CAD build for the part. Positions are in the model's coordinates, mm. Round coordinates to 2 decimals unless told otherwise and drop trailing zeros. Loops run counter-clockwise (first coordinate to the right, second up) from the corner with the lowest first, then second, coordinate; pieces in that order, holes last. Notation, with made-up numbers: M 41.25,27 L 81.25,27 A24 cw 81.25,37 Z; hole C 63.5,14 d10. An arc over 180 degrees is marked long. Use a Markdown table: item, result. Add a question column.
(1) Wall check: L1, parallel to Y at x = -8, z = 41; L2, parallel to Y at x = -8, z = 142.5; L3, parallel to X at y = -6, z = 482. Give the ranges that are in metal, low to high.
(2) Flat gauge pin, fed straight in: P1, Ø3, axis at x = 2, z = 545, coming from the +Y side. Where does the tip first touch, or does it go through?
(3) Band-saw the part on A-A, the plane z = 437.5. Write the cut outline in (x, y), and give its area (3 significant figures).
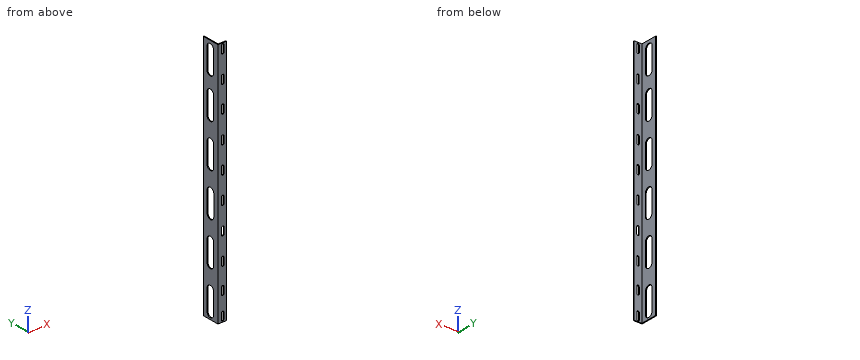
from build123d import *

# Parameters (mm, degrees)
BOSS_EXTRUDE1_DEPTH = 705
CUT_EXTRUDE2_DEPTH  = 10
CUT_EXTRUDE3_DEPTH  = 10


with BuildPart() as part:
    # Sketch1 → Boss-Extrude1 (new body)
    with BuildSketch(Plane.XY):
        Polygon((-9.451520251, 23.80952381), (-9.451520251, -26.19047619), (15.548479749, -26.19047619), (15.548479749, -23.69047619), (-6.951520251, -23.69047619), (-6.951520251, 23.80952381), align=None)
    extrude(amount=BOSS_EXTRUDE1_DEPTH)

    # Sketch3 → Cut-Extrude2 (cut)
    with BuildSketch(Plane(origin=(0, -23.69047619, 0), x_dir=(1, 0, 0), z_dir=(0, 1, 0))):
        with BuildLine():
            Line((1.100010518, -238.921557585), (1.100010518, -219.921557585))
            ThreePointArc((1.100010518, -219.921557585), (4.600010518, -217.057732255), (8.100010518, -219.921557585))
            Line((8.100010518, -219.921557585), (8.100010518, -238.921557585))
            ThreePointArc((8.100010518, -238.921557585), (4.600010518, -242.50349619), (1.100010518, -238.921557585))
        make_face()
        with BuildLine():
            Line((1.062751019, -162.814659823), (1.06366359, -143.814659845))
            ThreePointArc((1.06366359, -143.814659845), (4.564952106, -140.315948836), (8.063663115, -143.817237352))
            Line((8.063663115, -143.817237352), (8.064681771, -162.817237325))
            ThreePointArc((8.064681771, -162.817237325), (4.562374007, -166.462622847), (1.062751019, -162.814659823))
        make_face()
        with BuildLine():
            Line((0.583868221, -24.003598612), (0.583868221, -6.003598612))
            ThreePointArc((0.583868221, -6.003598612), (4.083868221, -2.503598612), (7.583868221, -6.003598612))
            Line((7.583868221, -6.003598612), (7.583868221, -24.003598612))
            ThreePointArc((7.583868221, -24.003598612), (4.083868221, -27.503598612), (0.583868221, -24.003598612))
        make_face()
        with BuildLine():
            Line((0.999318179, -316.46999614), (0.999318179, -297.46999614))
            ThreePointArc((0.999318179, -297.46999614), (4.499318179, -294.01841185), (7.999318179, -297.46999614))
            Line((7.999318179, -297.46999614), (7.999318179, -316.46999614))
            ThreePointArc((7.999318179, -316.46999614), (4.499318179, -320.051934745), (0.999318179, -316.46999614))
        make_face()
        with BuildLine():
            Line((0.793870885, -392.945206895), (0.793870885, -373.945206895))
            ThreePointArc((0.793870885, -373.945206895), (4.293870885, -370.493622604), (7.793870885, -373.945206895))
            Line((7.793870885, -373.945206895), (7.793870885, -392.945206895))
            ThreePointArc((7.793870885, -392.945206895), (4.293870885, -396.527145499), (0.793870885, -392.945206895))
        make_face()
        with BuildLine():
            Line((0.80674983, -468.976356015), (0.80674983, -449.976356015))
            ThreePointArc((0.80674983, -449.976356015), (4.30674983, -446.524771725), (7.80674983, -449.976356015))
            Line((7.80674983, -449.976356015), (7.80674983, -468.976356015))
            ThreePointArc((7.80674983, -468.976356015), (4.30674983, -472.55829462), (0.80674983, -468.976356015))
        make_face()
        with BuildLine():
            Line((0.838773895, -546.576842351), (0.838773895, -528.023898071))
            ThreePointArc((0.838773895, -528.023898071), (4.338773895, -524.572313781), (7.838773895, -528.023898071))
            Line((7.838773895, -528.023898071), (7.838773895, -546.576842351))
            ThreePointArc((7.838773895, -546.576842351), (4.338773895, -550.644510243), (0.838773895, -546.576842351))
        make_face()
        with BuildLine():
            Line((0.888336666, -621.781220279), (0.888336666, -602.781220279))
            ThreePointArc((0.888336666, -602.781220279), (4.388336666, -599.329635989), (7.888336666, -602.781220279))
            Line((7.888336666, -602.781220279), (7.888336666, -621.781220279))
            ThreePointArc((7.888336666, -621.781220279), (4.388336666, -625.363158884), (0.888336666, -621.781220279))
        make_face()
        with BuildLine():
            Line((0.754778841, -698.918998588), (0.754778841, -679.918998588))
            ThreePointArc((0.754778841, -679.918998588), (4.254778841, -676.361761205), (7.754778841, -679.918998588))
            Line((7.754778841, -679.918998588), (7.754778841, -698.918998588))
            ThreePointArc((7.754778841, -698.918998588), (4.254778841, -702.500937193), (0.754778841, -698.918998588))
        make_face()
        with BuildLine():
            Line((0.838792542, -89.065486865), (0.838792542, -70.065486865))
            ThreePointArc((0.838792542, -70.065486865), (4.338792542, -67.201661534), (7.838792542, -70.065486865))
            Line((7.838792542, -70.065486865), (7.838792542, -89.065486865))
            ThreePointArc((7.838792542, -89.065486865), (4.338792542, -92.647425469), (0.838792542, -89.065486865))
        make_face()
    extrude(amount=-CUT_EXTRUDE2_DEPTH, mode=Mode.SUBTRACT)

    # Sketch2 → Cut-Extrude3 (cut)
    with BuildSketch(Plane(origin=(-6.951520251, 0, 0), x_dir=(0, 0, -1), z_dir=(1, 0, 0))):
        with BuildLine():
            Line((-685.173208755, 11.86647277), (-626.275157977, 11.86647277))
            ThreePointArc((-626.275157977, 11.86647277), (-614.769492243, 0.360807036), (-626.275157977, -11.144858697))
            Line((-626.275157977, -11.144858697), (-685.173208755, -11.144858697))
            ThreePointArc((-685.173208755, -11.144858697), (-696.678874489, 0.360807036), (-685.173208755, 11.86647277))
        make_face()
        with BuildLine():
            Line((-570.642955191, 11.631729837), (-511.744904413, 11.631729837))
            ThreePointArc((-511.744904413, 11.631729837), (-500.239238679, 0.126064103), (-511.744904413, -11.379601631))
            Line((-511.744904413, -11.379601631), (-570.642955191, -11.379601631))
            ThreePointArc((-570.642955191, -11.379601631), (-582.148620925, 0.126064103), (-570.642955191, 11.631729837))
        make_face()
        with BuildLine():
            Line((-446.744904413, 11.34825395), (-387.846853634, 11.34825395))
            ThreePointArc((-387.846853634, 11.34825395), (-376.3411879, -0.157411783), (-387.846853634, -11.663077517))
            Line((-387.846853634, -11.663077517), (-446.744904413, -11.663077517))
            ThreePointArc((-446.744904413, -11.663077517), (-458.250570146, -0.157411783), (-446.744904413, 11.34825395))
        make_face()
        with BuildLine():
            Line((-322.846853634, 11.087774361), (-263.948802855, 11.087774361))
            ThreePointArc((-263.948802855, 11.087774361), (-252.615852555, -0.417891372), (-263.948802855, -11.923557106))
            Line((-263.948802855, -11.923557106), (-322.846853634, -11.923557106))
            ThreePointArc((-322.846853634, -11.923557106), (-334.352519367, -0.417891372), (-322.846853634, 11.087774361))
        make_face()
        with BuildLine():
            Line((-199.12283439, 11.260273997), (-140.224783611, 11.260273997))
            ThreePointArc((-140.224783611, 11.260273997), (-128.719117878, -0.245391736), (-140.224783611, -11.75105747))
            Line((-140.224783611, -11.75105747), (-199.12283439, -11.75105747))
            ThreePointArc((-199.12283439, -11.75105747), (-210.628500124, -0.245391736), (-199.12283439, 11.260273997))
        make_face()
        with BuildLine():
            Line((-75.224783611, 11.402162448), (-16.326732833, 11.402162448))
            ThreePointArc((-16.326732833, 11.402162448), (-4.821067099, -0.103503285), (-16.326732833, -11.609169019))
            Line((-16.326732833, -11.609169019), (-75.224783611, -11.609169019))
            ThreePointArc((-75.224783611, -11.609169019), (-86.730449345, -0.103503285), (-75.224783611, 11.402162448))
        make_face()
    extrude(amount=-CUT_EXTRUDE3_DEPTH, mode=Mode.SUBTRACT)


solid = part.part
Return value:
| question | item | result |
|---|---|---|
| 1 | L1 | -26.19 to -11.61, 11.4 to 23.81 |
| 1 | L2 | -26.19 to -11.75, 11.26 to 23.81 |
| 1 | L3 | -9.45 to -6.95 |
| 2 | P1 | y = -23.69 |
| 3 | outline | M -9.45,-26.19 L 15.55,-26.19 L 15.55,-23.69 L -6.95,-23.69 L -6.95,-11.66 L -9.45,-11.66 Z; M -9.45,11.35 L -6.95,11.35 L -6.95,23.81 L -9.45,23.81 Z |
| 3 | area | 124 mm^2 |
